from build123d import *

# Parameters (mm, degrees)
FLANGE_BASE1_START    = -3
FLANGE_BASE1_DEPTH    = 3
ESBO_O2_W             = 58.045623223
ESBO_O2_H             = 46
CORTE_EXTRUS_O1_DEPTH = 10
CORTE_EXTRUS_O2_START = -10
CORTE_EXTRUS_O2_DEPTH = 10


# Read off the part's stored shape, not the designer's step: Flange-base1
with BuildPart() as part:
    # Flange-base1 outline → Flange-base1 (new body)
    with BuildSketch(Plane.XY.offset(FLANGE_BASE1_START)):
        with BuildLine():
            ThreePointArc((-158.113883008, 56.35083269), (-250, 250), (-158.113883008, 443.64916731))
            Line((-158.113883008, 443.64916731), (-182.638577841, 443.64916731))
            ThreePointArc((-182.638577841, 443.64916731), (-227.927116936, 431.424151892), (-260.912254059, 398.070239015))
            ThreePointArc((-260.912254059, 398.070239015), (-300, 250), (-260.912254059, 101.929760985))
            ThreePointArc((-260.912254059, 101.929760985), (-227.927116936, 68.575848108), (-182.638577841, 56.35083269))
            Line((-182.638577841, 56.35083269), (-158.113883008, 56.35083269))
        make_face()
    extrude(amount=FLANGE_BASE1_DEPTH)

    # Esboço2 → Corte-extrusão1 (cut)
    with BuildSketch(Plane.XY):
        with Locations((-309.022811612, 184.35083269)):
            Rectangle(ESBO_O2_W, ESBO_O2_H)
    extrude(amount=-CORTE_EXTRUS_O1_DEPTH, mode=Mode.SUBTRACT)

    # Esboço3 → Corte-extrusão2 (cut)
    with BuildSketch(Plane.XY.offset(CORTE_EXTRUS_O2_START)):
        with BuildLine():
            Line((-160.011249605, 445.972957318), (-158.113883008, 443.64916731))
            ThreePointArc((-158.113883008, 443.64916731), (-250, 250), (-158.113883008, 56.35083269))
            Line((-158.113883008, 56.35083269), (-160.011249605, 54.027042682))
            ThreePointArc((-160.011249605, 54.027042682), (-253, 250), (-160.011249605, 445.972957318))
        make_face()
    extrude(amount=CORTE_EXTRUS_O2_DEPTH, mode=Mode.SUBTRACT)


solid = part.part
Work out the finished part from the listing and answer in its coordinate system (mm). Give positions to 0.01 mm unless a question says otherwise; leave off trailing zeros. Order: outer loops, then holes, each group sorted by start corner. A loop starts at its lowest first (then second) coordinate and runs counter-clockwise, first axis right, second up. Notation, with made-up numbers: (82.5, 29) -> (137.5, 29) arc R23 ccw to (137.5, 41) -> close; hole circle Ø4 at (63.25, 54). An arc over 180 degrees is marked (long way). One line per item, written item: value.
Item 1: Straight lines are drawn through the part: probe 1 along Y at (x, z) = (-188.5, -1.3); probe 2 along Y at (x, z) = (-198.5, -1.4); probe 3 along X at (y, z) = (278.5, -2). For each, find the intervals that lie inside material, in ascending order.
Answer sheet:
probe 1: 56.54 to 81.25, 418.75 to 443.46
probe 2: 57.76 to 93.13, 406.87 to 442.24
probe 3: -298.64 to -251.39
Item 2: Determine the mould class of faces 1 (the cylindrical face through (-228.5, 68.91, -1.52)), 2 (the flat face through (-262, 251, -3)), 3 (the cylindrical face through (-252.98, 246.91, -1.52)) for opening direction Y: released by +Y, released by -Y, zero draft, split by the parting line, or undercut.
Answer sheet:
face 1: released by -Y
face 2: zero draft
face 3: undercut
Item 3: Find section B-B, the plane z = -1.25. Give the vertices of the cut face in (x, y), plus the area to 3 significant figures.
Answer sheet:
outline: (-296.95, 207.35) -> (-280, 207.35) -> (-280, 161.35) -> (-286.6, 161.35) arc R300 ccw to (-260.91, 101.93) arc R90 ccw to (-182.64, 56.35) -> (-162.82, 56.35) arc R253 cw to (-162.82, 443.65) -> (-182.64, 443.65) arc R90 ccw to (-260.91, 398.07) arc R300 ccw to start
area: 18,900 mm²
Item 4: Flat-ended cylindrical pins translate along their axes: P1, Ø0.9, axis at y = 181.5, z = -1, coming from the -X side; P2, Ø1, axis at x = -238.5, z = -1.5, coming from the +Y side; P3, Ø1.5, axis at x = -289.5, z = -1.5, coming from the -Y side. Find the tip coordinate at first contact, or state that the pin passes through.
Answer sheet:
P1: x = -280
P2: y = 424.61
P3: y = 207.35
Item 5: Find section C-C, the plane x = -243.5. Give the vertices of the cut face in (y, z), plus the area to 3 significant figures.
Answer sheet:
outline: (80.05, -3) -> (181.32, -3) -> (181.32, 0) -> (80.05, 0) -> close; (318.68, -3) -> (419.95, -3) -> (419.95, 0) -> (318.68, 0) -> close
area: 608 mm²
Item 6: Find section D-D, the plane y = 349. Give the vertices of the cut face in (x, z), plus the area to 3 significant figures.
Answer sheet:
outline: (-283.19, -3) -> (-232.83, -3) -> (-232.83, 0) -> (-283.19, 0) -> close
area: 151 mm²
Item 7: Find section A-A, the plane x = -224. Give the vertices of the cut face in (y, z), plus the area to 3 significant figures.
Answer sheet:
outline: (66.42, -3) -> (132.39, -3) -> (132.39, 0) -> (66.42, 0) -> close; (367.61, -3) -> (433.58, -3) -> (433.58, 0) -> (367.61, 0) -> close
area: 396 mm²
